Work out the finished part from the listing and answer in its coordinate system (mm). A direction names the side the tool comes from. Coordinates: 2 decimals unless noted, no trailing zeros. Write each loop counter-clockwise with the first axis right and the second up, starting at its lowest first coordinate (ties: lowest second). Pieces come first, ordered by that corner, then holes. Notation, with made-up numbers: M -3,77.5 L 37,77.5 A29 ccw 37,99.5 Z; hole C 9.5,-14 d5. An arc over 180 degrees is marked long. Answer as CSV lines item,"result". Start each with the question number.
(1) A cutting plane is placed at D-D on z = -29. Give the vertices of the cut face in (x, y), then the cut area to 3 significant figures.
(2) Flat-ended cylindrical pins translate along their axes: P1, Ø1.3, axis at x = 9.5, y = 13.5, coming from the -Z side; P2, Ø1.8, axis at y = 6, z = -74.5, coming from the +X side; P3, Ø1.5, axis at x = 9.5, y = 17.5, coming from the +Z side; P4, Ø8, axis at y = 10.5, z = -41, coming from the +X side. Find the tip coordinate at first contact, or state that the pin passes through.
(3) For faces 5 (the flat face through (4, 13, -52)), 6 (the flat face through (8, 21, -109)), 7 (the flat face through (9, 13, -108.5)), 8 (the cylindrical face through (7.58, 14.34, 0.99)), determine the directions among +Z, -Z, +X, -X, +Y, -Y from which every point of the face is accessible in a straight line to the end or side of a thin tool.
(4) The mould has two halves that part along X. Classify faces 1 (the flat face through (17, 13, -107)), 2 (the flat face through (10, 19, -108)), 3 (the flat face through (8, 21, 3)), 4 (the flat face through (10, 7, -108)): released by +X, released by -X, zero draft, split by the parting line, or undercut.
(5) A cutting plane is placed at C-C on y = 6. Count the separate pieces of the cut face and the enclosed holes in it, then the cut area to 3 significant figures.
(6) A cutting plane is placed at A-A on z = -74.5. Give the vertices of the cut face in (x, y).
(7) Find the intervals of material crossed by L1, parallel to Z at x = 3.5, y = 6.25; L2, parallel to X at y = 21.25, z = -88; L3, parallel to Z at x = 3.25, y = 1.75, in increasing order. Write a range as [from, to].
from build123d import *

# Parameters (mm, degrees)
ESQUISSE1_W             = 17
ESQUISSE1_H             = 26
BOSS_EXTRU_1_DEPTH      = 3
ESQUISSE3_W             = 4
ESQUISSE3_H             = 26
BOSS_EXTRU_2_DEPTH      = 109
ESQUISSE4_R             = 1.5
ENL_V_MAT_EXTRU_2_DEPTH = 4
ESQUISSE5_R             = 1.5
ENL_V_MAT_EXTRU_3_DEPTH = 4
ESQUISSE6_W             = 3
ESQUISSE6_H             = 26
BOSS_EXTRU_3_DEPTH      = 13
ESQUISSE8_R             = 5.25
ENL_V_MAT_EXTRU_4_DEPTH = 2
ENL_V_START             = -2
ESQUISSE9_R             = 5.25
ENL_V_MAT_EXTRU_5_DEPTH = 2
ESQUISSE10_W            = 17
ESQUISSE10_H            = 4
BOSS_EXTRU_5_DEPTH      = 0.5
ESQUISSE11_W            = 17
ESQUISSE11_H            = 4.5
ENL_V_MAT_EXTRU_6_DEPTH = 0.5


with BuildPart() as part:
    # Esquisse1 → Boss.-Extru.1 (new body)
    with BuildSketch(Plane.XY):
        with Locations((8.5, 13)):
            Rectangle(ESQUISSE1_W, ESQUISSE1_H)
    extrude(amount=BOSS_EXTRU_1_DEPTH)

    # Esquisse3 → Boss.-Extru.2 (add)
    with BuildSketch(Plane(origin=(0, 0, 0), x_dir=(-1, 0, 0), z_dir=(0, 0, -1))):
        with Locations((-2, 13)):
            Rectangle(ESQUISSE3_W, ESQUISSE3_H)
    extrude(amount=BOSS_EXTRU_2_DEPTH)

    # Esquisse4 → Enlèv. mat.-Extru.2 (cut)
    with BuildSketch(Plane.ZY):
        with Locations((-8.5, 20)):
            Circle(ESQUISSE4_R)
        with Locations((-8.5, 6)):
            Circle(ESQUISSE4_R)
        with Locations((-26.496682549, 20)):
            Circle(ESQUISSE4_R)
        with Locations((-26.496682549, 6)):
            Circle(ESQUISSE4_R)
    extrude(amount=-ENL_V_MAT_EXTRU_2_DEPTH, mode=Mode.SUBTRACT)

    # Esquisse5 → Enlèv. mat.-Extru.3 (cut)
    with BuildSketch(Plane.ZY):
        with Locations((-92.5, 19.999545392)):
            Circle(ESQUISSE5_R)
        with Locations((-92.5, 6)):
            Circle(ESQUISSE5_R)
        with Locations((-74.5, 19.999545392)):
            Circle(ESQUISSE5_R)
        with Locations((-74.5, 6)):
            Circle(ESQUISSE5_R)
    extrude(amount=-ENL_V_MAT_EXTRU_3_DEPTH, mode=Mode.SUBTRACT)

    # Esquisse6 → Boss.-Extru.3 (add)
    with BuildSketch(Plane(origin=(4, 0, 0), x_dir=(0, 0, -1), z_dir=(1, 0, 0))):
        with Locations((107.5, 13)):
            Rectangle(ESQUISSE6_W, ESQUISSE6_H)
    extrude(amount=BOSS_EXTRU_3_DEPTH)

    # Esquisse8 → Enlèv. mat.-Extru.4 (cut)
    with BuildSketch(Plane(origin=(0, 0, 0), x_dir=(-1, 0, 0), z_dir=(0, 0, -1))):
        with Locations((-10, 7)):
            Circle(ESQUISSE8_R)
        with Locations((-10, 19)):
            Circle(ESQUISSE8_R)
    extrude(amount=-ENL_V_MAT_EXTRU_4_DEPTH, mode=Mode.SUBTRACT)

    # Esquisse9 → Enlèv. mat.-Extru.5 (cut)
    with BuildSketch(Plane.XY.offset(-106).offset(ENL_V_START)):
        with Locations(Location((10, 19, 0), (0, 0, 180))):
            Circle(ESQUISSE9_R)
        with Locations(Location((10, 7, 0), (0, 0, 180))):
            Circle(ESQUISSE9_R)
    extrude(amount=ENL_V_MAT_EXTRU_5_DEPTH, mode=Mode.SUBTRACT)

    # Esquisse10 → Boss.-Extru.5 (add)
    with BuildSketch(Plane.XY.offset(3)):
        with Locations((8.5, 13)):
            Rectangle(ESQUISSE10_W, ESQUISSE10_H)
    extrude(amount=BOSS_EXTRU_5_DEPTH)

    # Esquisse11 → Enlèv. mat.-Extru.6 (cut)
    with BuildSketch(Plane(origin=(0, 0, -109), x_dir=(-1, 0, 0), z_dir=(0, 0, -1))):
        with Locations((-8.5, 13)):
            Rectangle(ESQUISSE11_W, ESQUISSE11_H)
    extrude(amount=-ENL_V_MAT_EXTRU_6_DEPTH, mode=Mode.SUBTRACT)


solid = part.part
Here are the results:
1,outline,"M 0,0 L 4,0 L 4,26 L 0,26 Z"
1,area,"104 mm^2"
2,P1,"stops at z = -108.5"
2,P2,"passes through"
2,P3,"stops at z = 3"
2,P4,"stops at x = 4"
3,face 5,"+X, +Y, -Y"
3,face 6,"-Z, +X, -X, +Y, -Y"
3,face 7,"-Z, +X, -X"
3,face 8,"none"
4,face 1,"released by +X"
4,face 2,"undercut"
4,face 3,"zero draft"
4,face 4,"undercut"
5,separate pieces,"5"
5,enclosed holes,"0"
5,area,"437 mm^2"
6,outline,"M 0,0 L 4,0 L 4,4.5 L 0,4.5 Z; M 0,7.5 L 4,7.5 L 4,18.5 L 0,18.5 Z; M 0,21.5 L 4,21.5 L 4,26 L 0,26 Z"
7,L1,"z = [-109, -93.98], [-91.02, -75.98], [-73.02, -27.98], [-25.02, -9.98], [-7.02, 3]"
7,L2,"x = [0, 4]"
7,L3,"z = [-109, 3]"
